Work out the finished part from the listing and answer in its coordinate system (mm). A direction names the side the tool comes from. Give positions to 0.01 mm unless a question says otherwise; leave off trailing zeros. Loops run counter-clockwise (first coordinate to the right, second up) from the corner with the lowest first, then second, coordinate; pieces in that order, holes last. Notation, with made-up numbers: M 80.25,-4 L 117.25,-4 A23 cw 117.25,22 Z; hole C 56.5,20 d6. An arc over 180 degrees is marked long. Answer as a JSON object with one key per item and string values. Group by question number.
```python
from build123d import *

# Parameters (mm, degrees)
BOSS_EXTRUDE1_DEPTH = 2.75
CUT_EXTRUDE1_DEPTH  = 3
SKETCH3_R           = 0.5
CUT_EXTRUDE2_DEPTH  = 1.25
CUT_EXTRUDE3_START  = 17.5
CUT_EXTRUDE3_DEPTH  = 12.5
SKETCH5_W           = 14.8
SKETCH5_H           = 2.5
CUT_EXTRUDE4_DEPTH  = 36.5
CUT_EXTRUDE5_START  = 35.5
CUT_EXTRUDE5_DEPTH  = 13.5
SKETCH7_R           = 0.5
CUT_EXTRUDE6_DEPTH  = 3
CUT_EXTRUDE7_REACH  = 62.5
SKETCH8_R           = 1


with BuildPart() as part:
    # Sketch1 → Boss-Extrude1 (new body, symmetric)
    with BuildSketch(Plane.XY):
        with BuildLine():
            Line((0, 0), (0, 12.5))
            Line((0, 12.5), (-61.5, 12.5))
            ThreePointArc((-61.5, 12.5), (-62.560660172, 12.939339828), (-63, 14))
            Line((-63, 14), (-63, 16.693487943))
            ThreePointArc((-63, 16.693487943), (-62.853553391, 17.047041334), (-62.5, 17.193487943))
            Line((-62.5, 17.193487943), (-62, 17.193487943))
            Line((-62, 17.193487943), (-62, 29.193487943))
            ThreePointArc((-62, 29.193487943), (-67.10498068, 22.897467949), (-68.93, 15))
            Line((-68.93, 15), (-68.93, -3))
            Line((-68.93, -3), (-54, -3))
            Line((-54, -3), (-54, -19.2))
            Line((-54, -19.2), (-54.8, -20))
            Line((-54.8, -20), (-54.8, -48))
            Line((-54.8, -48), (-48.67612206, -44.87972834))
            Line((-48.67612206, -44.87972834), (-40, -12.5))
            Line((-40, -12.5), (0, -12.5))
            Line((0, -12.5), (0, 0))
        make_face()
    extrude(amount=BOSS_EXTRUDE1_DEPTH, both=True)

    # Sketch2 → Cut-Extrude1 (cut)
    with BuildSketch(Plane.XY.offset(2.75)):
        Polygon((0, -8), (-54, -8), (-84.556927157, -8), (-84.556927157, 35.37162012), (-54, 35.37162012), (-54, 8), (0, 8), align=None)
    extrude(amount=-CUT_EXTRUDE1_DEPTH, mode=Mode.SUBTRACT)

    # Sketch3 → Cut-Extrude2 (cut)
    with BuildSketch(Plane.XY.offset(2.75)):
        with Locations((-4, 11)):
            Circle(SKETCH3_R)
        with Locations((-27, 11)):
            Circle(SKETCH3_R)
        with Locations((-50, 11)):
            Circle(SKETCH3_R)
        with Locations((-50, -11)):
            Circle(SKETCH3_R)
        with Locations((-27, -11)):
            Circle(SKETCH3_R)
        with Locations((-4, -11)):
            Circle(SKETCH3_R)
    extrude(amount=-CUT_EXTRUDE2_DEPTH, mode=Mode.SUBTRACT)

    # Sketch4 → Cut-Extrude3 (cut)
    with BuildSketch(Plane(origin=(0, 12.5, 0), x_dir=(1, 0, 0), z_dir=(0, 1, 0)).offset(CUT_EXTRUDE3_START)):
        Polygon((-68.93, 2.75), (-62, 0.5), (-62, 2.75), align=None)
    extrude(amount=-CUT_EXTRUDE3_DEPTH, mode=Mode.SUBTRACT)

    # Sketch5 → Cut-Extrude4 (cut, through all)
    with BuildSketch(Plane.XZ.offset(12.5)):
        with Locations((-47.4, -1.5)):
            Rectangle(SKETCH5_W, SKETCH5_H)
    extrude(amount=CUT_EXTRUDE4_DEPTH, mode=Mode.SUBTRACT)

    # Sketch6 → Cut-Extrude5 (cut)
    with BuildSketch(Plane.XZ.offset(12.5).offset(CUT_EXTRUDE5_START)):
        Polygon((-54.8, 2.75), (-54.8, 0.25), (-49.674240396, 2.75), align=None)
    extrude(amount=-CUT_EXTRUDE5_DEPTH, mode=Mode.SUBTRACT)

    # Sketch7 → Cut-Extrude6 (cut)
    with BuildSketch(Plane(origin=(0, 12.5, 0), x_dir=(1, 0, 0), z_dir=(0, 1, 0))):
        with Locations((-7.54, -1.25)):
            Circle(SKETCH7_R)
        with Locations((-48.34, -1.25)):
            Circle(SKETCH7_R)
    extrude(amount=-CUT_EXTRUDE6_DEPTH, mode=Mode.SUBTRACT)

    # Sketch8 → Cut-Extrude7 (cut, up to next)
    with BuildSketch(Plane(origin=(0, 12.5, 0), x_dir=(1, 0, 0), z_dir=(0, 1, 0)), mode=Mode.PRIVATE) as cut_extrude7_sk1:
        with Locations((-27.94, -1.25)):
            Circle(SKETCH8_R)
    cut_extrude7_tool1 = extrude(cut_extrude7_sk1.sketch, amount=-CUT_EXTRUDE7_REACH, mode=Mode.PRIVATE) & part.part
    add(cut_extrude7_tool1.solids().sort_by_distance((-27.94, 12.5, 1.25))[0], mode=Mode.SUBTRACT)


solid = part.part
```
Item 1: Given pin 1 Ø0.9 at (y, z) = (-33, 1.5) entering from -X; pin 2 Ø0.8 at (x, y) = (-4, 11) entering from +Z; pin 3 Ø16.5 at (x, y) = (-48, -35) entering from -Z; pin 4 Ø11 at (x, y) = (-21, 18.5) entering from +Z, each flat-ended and moving along its own axis, determine where each tip first touches the part or whether it passes through.
Item 2: A cutting plane is placed at A-A (x = -21). Determine the outline of the cut face in (y, z), and give its area (3 significant figures).
Item 3: Find the intervals of material crossed by probe 1 along Y at (x, z) = (-32, 1.15); probe 2 along Y at (x, z) = (-27, 2.15); probe 3 along Z at (x, y) = (-27.94, 9.5), in increasing order. Write a range as [from, to].
Item 4: A cutting plane is placed at C-C (y = -42). Determine the outline of the cut face in (x, z).
Item 5: A tool of negligible diameter and unlimited length cuts with its end or side. For faces 1 (the flat face through (-53, -34.5, 2)), 2 (the flat face through (-62, -3, -1)), 3 (the flat face through (-49, -26, -0.25)), from which of +Z, -Z, +X, -X, +Y, -Y can it reach the whole face along a straight path? Write none if from no direction.
Item 6: For a pull along Y with two mould halves and no side action, classify faces 4 (the flat face through (-63, 15, -1)), 5 (the flat face through (-51.1, -46.115, 0.938)), 6 (the flat face through (-64.674, 22.129, -1.368)) as pulls with the +Y half, pulls with the -Y half, needs draft (parallel to the pull), parting line crosses it, or undercut.
Item 7: A cutting plane is placed at D-D (y = -31). Determine the outline of the cut face in (x, z).
Item 8: A cutting plane is placed at B-B (z = -1.8). Determine the outline of the cut face in (x, y).
The answers:
{
 "1": {"pin 1": "stops at x = -54.8", "pin 2": "stops at z = 1.5", "pin 3": "stops at z = -0.25", "pin 4": "passes through"},
 "2": {"outline": "M -12.5,-2.75 L 12.5,-2.75 L 12.5,2.75 L 8,2.75 L 8,-0.25 L -8,-0.25 L -8,2.75 L -12.5,2.75 Z", "area": "89.5 mm^2"},
 "3": {"probe 1": "y = [-12.5, -8], [8, 12.5]", "probe 2": "y = [-12.5, -11.5], [-10.5, -8], [8, 10.5], [11.5, 12.5]", "probe 3": "z = [-2.75, 0.25], [2.25, 2.75]"},
 "4": {"outline": "M -54.8,-0.25 L -47.9,-0.25 L -47.9,2.75 L -49.67,2.75 L -54.8,0.25 Z"},
 "5": {"face 1": "+Z, -X, -Y", "face 2": "+Z, -Z, -X, -Y", "face 3": "-Z, +X, -X, -Y"},
 "6": {"face 4": "undercut", "face 5": "pulls with the -Y half", "face 6": "needs draft"},
 "7": {"outline": "M -54.8,-0.25 L -44.96,-0.25 L -44.96,2.75 L -54.8,2.75 Z"},
 "8": {"outline": "M -68.93,-3 L -54,-3 L -54,-12.5 L 0,-12.5 L 0,12.5 L -61.5,12.5 A1.5 cw -63,14 L -63,16.69 A0.5 cw -62.5,17.19 L -62,17.19 L -62,17.5 L -66,17.5 L -66,24.84 A18 ccw -68.93,15 Z"}
}
